```python
from build123d import *

# Parameters (mm, degrees)
F1_DEPTH = 82.55
F2_R     = 20.6375
F3_DEPTH = 12.7
F5_DEPTH = 25.4
F6_R     = 23.8125
F7_DEPTH = 25.4


with BuildPart() as f1:
    # F0 (on Front) → F1 (new body)
    with BuildSketch(Plane.XZ):
        Polygon((0, 139.7), (0, 0), (190.5, 0), (190.5, 12.7), (25.4, 12.7), (25.4, 139.7), align=None)
    extrude(amount=F1_DEPTH)

    # F2 (on face) → F3 (cut, through all)
    with BuildSketch(Plane.XY.offset(12.7)):
        with Locations((76.2, -41.275)):
            Circle(F2_R)
        with Locations((152.4, -41.275)):
            Circle(F2_R)
    extrude(amount=-F3_DEPTH, mode=Mode.SUBTRACT)

    # F4 (on face) → F5 (cut)
    with BuildSketch(Plane(origin=(0, 0, 0), x_dir=(0, -1, 0), z_dir=(-1, 0, 0))):
        with BuildLine():
            ThreePointArc((0, 57.15), (41.275, 98.425), (82.55, 57.15))
            Line((82.55, 57.15), (82.55, 139.7))
            Line((82.55, 139.7), (0, 139.7))
            Line((0, 139.7), (0, 57.15))
        make_face()
    extrude(amount=-F5_DEPTH, mode=Mode.SUBTRACT)

    # F6 (on face) → F7 (cut, through all)
    with BuildSketch(Plane(origin=(0, 0, 0), x_dir=(0, -1, 0), z_dir=(-1, 0, 0))):
        with Locations((41.275, 57.15)):
            Circle(F6_R)
    extrude(amount=-F7_DEPTH, mode=Mode.SUBTRACT)


solid = f1.part
```
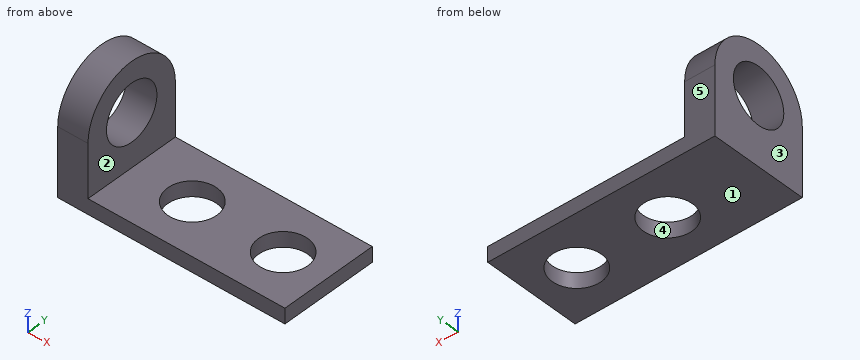
Geometry: final body of the model. Coordinates: model frame, mm. Face numbers are marked on the shaded views. A direction names the side the tool comes from. Coordinates: 2 decimals unless noted, no trailing zeros. Loops run counter-clockwise (first coordinate to the right, second up) from the corner with the lowest first, then second, coordinate; pieces in that order, holes last. Notation, with made-up numbers: (31, -2) -> (51, -2) arc R6 cw to (51, 9) -> close; hole circle Ø5 at (-14, 25.25). An arc over 180 degrees is marked (long way). Use a Markdown table: item, result. Add a question column.
(1) Section query B-B, the plane y = -60. Return loops of the section in (x, z), plus the area to 3 significant figures.
(2) Mould query, pull axis Y, two halves, no side actions, for the marked faces 3, 4 and 5. Classes: pulls with the +Y half, pulls with the -Y half, needs draft (parallel to the pull), parting line crosses it, or undercut.
(3) Section query A-A, the plane x = 152.4. Return loops of the section in (y, z), plus the area to 3 significant figures.
(4) Line query: line 1 along Y through (x, z) = (152.4, 4); line 2 along Z through (x, y) = (53.5, -69.5); line 3 along X through (y, z) = (-58.5, 78). Output: solid intervals per line, ascending.
(5) Access query for the marked faces 1 and 2. Directions: +Z, -Z, +X, -X, +Y, -Y. A direction counts if a zero-diameter tool reaches every point of the face in a straight line with its end or side. Return the directions, or none.
(6) Section query C-C, the plane z = 44.5. Return loops of the section in (x, y).
(7) Pin query (flat end, axial travel): pin 1 Ø2 at (y, z) = (-64.5, 25) entering from +X; pin 2 Ø6 at (x, y) = (110, -67) entering from +Z; pin 3 Ø8 at (y, z) = (-27.5, 79.5) entering from -X. Return the tip coordinate at first contact, or that it passes through.
(8) Section query D-D, the plane y = -35.5. Return loops of the section in (x, z).
Answer:
| question | item | result |
|---|---|---|
| 1 | outline | (0, 0) -> (67.52, 0) -> (67.52, 12.7) -> (25.4, 12.7) -> (25.4, 42.44) -> (0, 42.44) -> close; (0, 71.86) -> (25.4, 71.86) -> (25.4, 93.93) -> (0, 93.93) -> close; (84.88, 0) -> (143.72, 0) -> (143.72, 12.7) -> (84.88, 12.7) -> close; (161.08, 0) -> (190.5, 0) -> (190.5, 12.7) -> (161.08, 12.7) -> close |
| 1 | area | 3,290 mm^2 |
| 2 | face 3 | needs draft |
| 2 | face 4 | undercut |
| 2 | face 5 | pulls with the +Y half |
| 3 | outline | (-82.55, 0) -> (-61.91, 0) -> (-61.91, 12.7) -> (-82.55, 12.7) -> close; (-20.64, 0) -> (0, 0) -> (0, 12.7) -> (-20.64, 12.7) -> close |
| 3 | area | 524 mm^2 |
| 4 | line 1 | y = -82.55 to -61.91, -20.64 to 0 |
| 4 | line 2 | z = 0 to 12.7 |
| 4 | line 3 | x = 0 to 25.4 |
| 5 | face 1 | -Z, +X, -X, +Y, -Y |
| 5 | face 2 | +Z, +X, +Y, -Y |
| 6 | outline | (0, -82.55) -> (25.4, -82.55) -> (25.4, -61.45) -> (0, -61.45) -> close; (0, -21.1) -> (25.4, -21.1) -> (25.4, 0) -> (0, 0) -> close |
| 7 | pin 1 | stops at x = 25.4 |
| 7 | pin 2 | stops at z = 12.7 |
| 7 | pin 3 | stops at x = 0 |
| 8 | outline | (0, 0) -> (56.39, 0) -> (56.39, 12.7) -> (25.4, 12.7) -> (25.4, 34.05) -> (0, 34.05) -> close; (0, 80.25) -> (25.4, 80.25) -> (25.4, 98.02) -> (0, 98.02) -> close; (96.01, 0) -> (132.59, 0) -> (132.59, 12.7) -> (96.01, 12.7) -> close; (172.21, 0) -> (190.5, 0) -> (190.5, 12.7) -> (172.21, 12.7) -> close |
